Build history of the part. All positions in model axes, mm. A direction names the side the tool comes from. Round coordinates to 2 decimals unless told otherwise and drop trailing zeros. Write each loop counter-clockwise with the first axis right and the second up, starting at its lowest first coordinate (ties: lowest second). Pieces come first, ordered by that corner, then holes.
1) Saw through at B-B (y = 22). Write the cut outline in (x, z).
2) Saw through at C-C (z = 7.75). Write the cut outline in (x, y), plus the area to 3 significant figures.
3) Flat gauge pins, fed straight in: pin 1 (6 mm diameter, centred on x = 16.5, y = 15, fed in from -Z); pin 2 (3 mm diameter, centred on x = -15.5, z = 12.5, fed in from -Y); pin 3 (3.5 mm diameter, centred on y = 17.5, z = 5.5, fed in from -X); pin 4 (2 mm diameter, centred on y = -1, z = 13.5, fed in from -X). Where does each tip first touch, or does it go through?
4) Saw through at D-D (y = -4). Write the cut outline in (x, z).
5) Saw through at A-A (x = -17.8). Write the cut outline in (y, z).
6) Pull direction Z, two halves, no side cores. Call faces 4 (the flat face through (-20, 7.75, 8)), 5 (the flat face through (-13, 26.3, 8)), 6 (the flat face through (12, 12, 15.6)): +Z half, -Z half, draft (parallel to the pull), parting line (faces both ways), or undercut.
7) Which spindle directions (+Z, -Z, +X, -X, +Y, -Y) get a long thin tool onto all of the face, cutting with end or side? Do faces 1 (the cylindrical face through (25.035, 8.06, 7.691)), 2 (the cylindrical face through (6.4, 25.51, 7.69)), 3 (the flat face through (-18, 16, 14.3)). Say none if no direction does.
8) Wall check: probe 1 along Y at (x, z) = (-17.8, 9.25); probe 2 along Y at (x, z) = (0, 6); probe 3 along Z at (x, y) = (-12, 21.5). Give the ranges that are in metal, low to high.
Autodesk Inventor part; units mm, degrees
ref_plane "YZ Plane" through (0, 0, 0) normal (1, 0, 0) x (0, 1, 0)
ref_plane "XZ Plane" through (0, 0, 0) normal (0, 1, 0) x (-1, 0, 0)
ref_plane "XY Plane" through (0, 0, 0) normal (0, 0, 1) x (1, 0, 0)
sketch "Sketch1" plane through (0, 0, 0) normal (0, 0, 1) x (1, 0, 0)
  line L0 (-25.6, 26.3) -> (-25.6, 6.6)
  line L1 (-25.6, 26.3) -> (0, 26.3)
  line L2 (0, 26.3) -> (0, 0) construction
  line L3 (0, 0) -> (26.3, 0)
  arc A0 (26.3, 0) -> (21.4915, 15.1594) centre (0, 0) ccw
  line L4 (-25.6, 6.6) -> (-23.6, 6.6)
  circle A1 centre (-17.8, -20.3) radius 2.25
  arc A2 (0.8, -25.5) -> (26.3, 0) centre (0.8, 0) ccw
  line L5 (-6.4086, -25.5) -> (23, -25.5) construction
  arc A3 (-22.1547, 4.6986) -> (-23.6, 6.6) centre (-23.6, 5.1) ccw
  circle A4 centre (20.3, 22.8) radius 2.25
  arc A5 (-22.1547, 4.6986) -> (-19.151, -14.6964) centre (0.8, -1.6765) ccw
  arc A6 (-19.7128, -17.3689) -> (-19.151, -14.6964) centre (-20.7682, -15.7518) ccw
  arc A7 (-12.1947, -21.6439) -> (-14.8665, -22.2091) centre (-13.248, -23.2624) ccw
  arc A8 (-19.7128, -17.3689) -> (-14.8665, -22.2091) centre (-17.8, -20.3) ccw
  arc A9 (-12.1947, -21.6439) -> (0.8, -25.5) centre (0.8, -1.6765) ccw
  arc A10 (22.3174, 19.9399) -> (17.2258, 24.4732) centre (20.3, 22.8) ccw
  arc A11 (12.5728, 23.1001) -> (17.2258, 24.4732) centre (14.2128, 26.1131) ccw
  arc A12 (22.3174, 19.9399) -> (21.4915, 15.1594) centre (24.2947, 17.1367) ccw
  arc A13 (12.5728, 23.1001) -> (0, 26.3) centre (0, 0) ccw
  dimension "d1" = 25.6
  dimension "d2" = 19.7
  dimension "d6" = 4.5
  dimension "d8" = 17.8
  dimension "d9" = 26.3
  dimension "d10" = 51.8
  dimension "d11" = 20.3
  dimension "d12" = 1.5
  dimension "d13" = 4.5
  dimension "d14" = 22.8
  dimension "d15" = 20.3
  dimension "d16" = 2
  dimension "d18" = 90
  dimension "d19" = 90
  dimension "d20" = 1.25
  dimension "d21" = 1.25
  dimension "d22" = 90
  dimension "d23" = 90
extrude "Extrusion1" add sketch "Sketch1" along normal blind 15.6
sketch "Sketch2" plane through (-25.6, 6.6, 0) normal (-1, 0, 0) x (0, 0, 1)
  line L0 (1.7, 18.25) -> (14.3, 18.25)
  line L1 (14.3, 18.25) -> (14.3, 1.15)
  line L2 (14.3, 1.15) -> (1.7, 1.15)
  line L3 (1.7, 1.15) -> (1.7, 18.25)
  point P0 (0, -6.6)
  point P1 (0, 19.7)
  dimension "d26" = 12.6
  dimension "d27" = 17.1
  dimension "d28" = 1.7
  dimension "d29" = 1.45
extrude "Extrusion2" cut sketch "Sketch2" against normal blind 15.6
sketch "Sketch3" plane through (0, 0, 15.6) normal (0, 0, 1) x (1, 0, 0)
  circle A0 centre (0, 0) radius 16
  dimension "d32" = 32
extrude "Extrusion3" cut sketch "Sketch3" against normal blind 13.9
properties part number "5015 RADIAL FAN" material "PBT Plastic"
Evaluation:
1. outline: (-25.6, 0) - (18.2, 0) - (18.2, 15.6) - (-25.6, 15.6) - (-25.6, 14.3) - (-10, 14.3) - (-10, 1.7) - (-25.6, 1.7) - close; (22.4, 0) - (23.71, 0) - (23.71, 15.6) - (22.4, 15.6) - close
2. outline: (-25.6, 6.6) - (-23.6, 6.6) arc R1.5 cw to (-22.15, 4.7) arc R23.82 ccw to (-19.15, -14.7) arc R1.93 cw to (-19.71, -17.37) arc R3.5 ccw (long way) to (-14.87, -22.21) arc R1.93 cw to (-12.19, -21.64) arc R23.82 ccw to (0.8, -25.5) arc R25.5 ccw to (26.3, 0) arc R26.3 ccw to (21.49, 15.16) arc R3.43 cw to (22.32, 19.94) arc R3.5 ccw (long way) to (17.23, 24.47) arc R3.43 cw to (12.57, 23.1) arc R26.3 ccw to (0, 26.3) - (-25.6, 26.3) - (-25.6, 24.85) - (-10, 24.85) - (-10, 12.49) arc R16 cw (long way) to (-14, 7.75) - (-25.6, 7.75) - close; hole circle Ø4.5 at (-17.8, -20.3); hole circle Ø4.5 at (20.3, 22.8)
2. area: 1,190 mm2
3. pin 1: stops at z = 0
3. pin 2: stops at y = -23.71
3. pin 3: stops at x = -10
3. pin 4: stops at x = -23.02
4. outline: (-22.91, 0) - (25.98, 0) - (25.98, 15.6) - (15.49, 15.6) - (15.49, 1.7) - (-15.49, 1.7) - (-15.49, 15.6) - (-22.91, 15.6) - close
5. outline: (-23.8, 0) - (-22.55, 0) - (-22.55, 15.6) - (-23.8, 15.6) - close; (-18.05, 0) - (26.3, 0) - (26.3, 15.6) - (-18.05, 15.6) - close; hole (7.75, 1.7) - (24.85, 1.7) - (24.85, 14.3) - (7.75, 14.3) - close
6. face 4: undercut
6. face 5: draft
6. face 6: +Z half
7. face 1: +Z, -Z, +X
7. face 2: +Z, -Z, +Y
7. face 3: -X
8. probe 1: y = -23.8 to -22.55, -18.05 to 7.75, 24.85 to 26.3
8. probe 2: y = -25.49 to -16, 16 to 26.3
8. probe 3: z = 0 to 1.7, 14.3 to 15.6
